Here's how the part is built. I have some questions about the finished solid (model axes, mm). A direction names the side the tool comes from. Round coordinates to 2 decimals unless told otherwise and drop trailing zeros. Loops run counter-clockwise (first coordinate to the right, second up) from the corner with the lowest first, then second, coordinate; pieces in that order, holes last. Notation, with made-up numbers: (-32, 38.5) -> (12, 38.5) arc R21 cw to (12, 64.5) -> close; hole circle Ø9 at (35.25, 25.5). An arc over 180 degrees is marked (long way). Use one line per item in the form item = value. Start each with the question number.
Item 1: If we section it at D-D (x = 25.5): Write out the boundary of the cut face in (y, z).
Item 2: Thinking about a two-plate mould opening in Z: for faces 4 (the face through (-11.265, 97.072, 2.556)), 5 (the face through (-0.2, -0.4, 10.16)), 6 (the face through (-3, 0, 0)), which applies, released by +Z, released by -Z, zero draft, split by the parting line, or undercut?
Item 3: If we section it at C-C (y = -102.5): Write out the boundary of the cut face in (x, z) (3 decimals).
Item 4: For faces 1 (the face through (0, 82.55, 4)), 2 (the face through (0, 0, 8)), 3 (the face through (-28.49, 1.58, 5.01)), which set-ups out of +Z, -Z, +X, -X, +Y, -Y let a thin tool reach every point of the face, with its end or its side?
Item 5: If I drill on L1, parallel to Y at x = -4, z = 8.75; L2, parallel to X at y = 23, z = 5.5; L3, parallel to X at y = 86, z = 7, over which ranges is the centre line in solid material (lowest first)? Write a range as [from, to].
Item 6: If we section it at B-B (y = 76): Write out the boundary of the cut face in (x, z).
Item 7: If we section it at A-A (x = -3): Write out the boundary of the cut face in (y, z) (3 decimals), then the cut area to 3 significant figures.
Item 8: I'm going to push flat-ended pins straight in: pin 1 Ø0.9 at (x, y) = (-2, 89.5) entering from +Z; pin 2 Ø0.6 at (y, z) = (89.5, 2.5) entering from +X; pin 3 Ø16 at (x, y) = (-3, 38) entering from +Z; pin 4 Ø5 at (y, z) = (-54.5, 8) entering from -X. Where does each tip first touch, or does it pass through?
```python
from build123d import *

# Parameters (mm, degrees)
F1_DEPTH     = 7.62
F2_W         = 26.67
F2_H         = 5.08
F3_DEPTH     = 0.508
F5_DEPTH     = 7.62
F7_DEPTH     = 25.4
F8_T1_DEPTH  = 39.5884897473
F8_T3_DEPTH  = 43.1891092466
F8_T5_DEPTH  = 15.7316119842
F8_T10_DEPTH = 21.2484768612
F8_T15_DEPTH = 21.2484768612
F8_T20_DEPTH = 21.2484768612
F8_T25_DEPTH = 21.2484768612
F10_DEPTH    = 10.16
F12_DEPTH    = 3.175
F13_C1_SIZE2 = 5.08
F13_C1_SIZE  = 2.54
F13_C2_SIZE2 = 2.54
F13_C2_SIZE  = 5.08


# Not quite as in the source:
# - a fillet or chamfer that OpenCascade refuses, or shapes differently, is made with other operations: its cross-section is extruded or revolved along the edge and cut away or added


with BuildPart() as f1:
    # F0 (on Top) → F1 (new body)
    with BuildSketch(Plane.XY):
        Polygon((-15.875, 88.9), (-12.7, 0), (12.7, 0), (15.875, 88.9), align=None)
        Polygon((-6.5727372599, 6.35), (-9.2941658314, 82.55), (9.2941658314, 82.55), (6.5727372599, 6.35), align=None, mode=Mode.SUBTRACT)
    extrude(amount=F1_DEPTH)

    # F2 (on face) → F3 (join)
    with BuildSketch(Plane(origin=(0, 88.9, 0), x_dir=(-1, 0, 0), z_dir=(0, 1, 0))):
        with Locations((0, 2.54)):
            Rectangle(F2_W, F2_H)
    extrude(amount=F3_DEPTH)

    # F4 (on Top) → F5 (join, through all)
    with BuildSketch(Plane.XY):
        Polygon((-6.35, 105.2430003945), (-15.875, 89.408), (15.875, 89.408), (6.35, 105.2430003945), align=None)
    extrude(amount=F5_DEPTH)

    # F6 (on Right) → F7 (cut, symmetric)
    with BuildSketch(Plane.YZ):
        Polygon((105.2430003945, 7.62), (89.408, 7.62), (105.2430003945, 1.27), align=None)
    extrude(amount=F7_DEPTH, both=True, mode=Mode.SUBTRACT)

    # F8: chamfer of 1.524 on 6 edges, made by hand

    # F8_s2 → F8_t1 (cut)
    with BuildSketch(Plane.YZ.offset(-19.7942448737)):
        Polygon((88.9, 6.096), (87.376, 7.62), (88.9, 7.62), align=None)
    extrude(amount=F8_T1_DEPTH, mode=Mode.SUBTRACT)

    # F8_s4 → F8_t3 (cut)
    with BuildSketch(Plane.YZ.offset(-21.5945546233)):
        Polygon((89.408, 5.3668893881), (91.4992312711, 6.7813944907), (89.408, 7.62), align=None)
    extrude(amount=F8_T3_DEPTH, mode=Mode.SUBTRACT)

    # F8_s6 → F8_t5 (cut)
    with BuildSketch(Plane.XY.offset(-4.0558059921)):
        Polygon((14.2955997995, 88.9), (15.8186287896, 87.3216061075), (15.875, 88.9), align=None)
        Polygon((-14.2955997995, 88.9), (-15.8186287896, 87.3216061075), (-15.875, 88.9), align=None)
    extrude(amount=F8_T5_DEPTH, mode=Mode.SUBTRACT)


with BuildPart() as f8_tool8:
    # F8_s9 → F8_t10 (new body)
    with BuildSketch(Plane.XY.offset(-6.8142384306)):
        Polygon((13.1798265815, 89.408), (14.4857717649, 91.7175464201), (15.875, 89.408), align=None)
    extrude(amount=F8_T10_DEPTH)

    split(bisect_by=Plane.YZ.offset(13.335), keep=Keep.TOP)


with BuildPart() as f1_1:
    add(f1.part)

    # F8_t7: cut F8_tool8
    add(f8_tool8.part, mode=Mode.SUBTRACT)


with BuildPart() as f8_tool13:
    # F8_s14 → F8_t15 (new body)
    with BuildSketch(Plane.XY.offset(-6.8142384306)):
        Polygon((13.1798265815, 89.408), (14.4857717649, 91.7175464201), (15.875, 89.408), align=None)
    extrude(amount=F8_T15_DEPTH)

    split(bisect_by=Plane.XY.offset(5.08), keep=Keep.TOP)


with BuildPart() as f1_2:
    add(f1_1.part)

    # F8_t12: cut F8_tool13
    add(f8_tool13.part, mode=Mode.SUBTRACT)


with BuildPart() as f8_tool18:
    # F8_s19 → F8_t20 (new body)
    with BuildSketch(Plane.XY.offset(-6.8142384306)):
        Polygon((-14.4857717649, 91.7175464201), (-13.1798265815, 89.408), (-15.875, 89.408), align=None)
    extrude(amount=F8_T20_DEPTH)

    split(bisect_by=Plane.YZ.offset(-13.335), keep=Keep.BOTTOM)


with BuildPart() as f1_3:
    add(f1_2.part)

    # F8_t17: cut F8_tool18
    add(f8_tool18.part, mode=Mode.SUBTRACT)


with BuildPart() as f8_tool23:
    # F8_s24 → F8_t25 (new body)
    with BuildSketch(Plane.XY.offset(-6.8142384306)):
        Polygon((-14.4857717649, 91.7175464201), (-13.1798265815, 89.408), (-15.875, 89.408), align=None)
    extrude(amount=F8_T25_DEPTH)

    split(bisect_by=Plane.XY.offset(5.08), keep=Keep.TOP)


with BuildPart() as f1_4:
    add(f1_3.part)

    # F8_t22: cut F8_tool23
    add(f8_tool23.part, mode=Mode.SUBTRACT)

    # F9 (on Top) → F10 (join)
    with BuildSketch(Plane.XY):
        with BuildLine():
            Line((22.2250049976, 0), (-22.2250049976, 0))
            ThreePointArc((-22.2250049976, 0), (-28.5750049976, 1.626602675), (-33.360963964, 6.1057692308))
            Line((-33.360963964, 6.1057692308), (-35.0741884204, 5.0131183432))
            ThreePointArc((-35.0741884204, 5.0131183432), (-29.5519258835, -0.155151961), (-22.225, -2.032))
            Line((-22.225, -2.032), (22.225, -2.032))
            ThreePointArc((22.225, -2.032), (29.5519258835, -0.155151961), (35.0741884204, 5.0131183432))
            Line((35.0741884204, 5.0131183432), (33.360963964, 6.1057692308))
            ThreePointArc((33.360963964, 6.1057692308), (28.5750049976, 1.626602675), (22.2250049976, 0))
        make_face()
    extrude(amount=F10_DEPTH)

    # F11 (on Top) → F12 (join)
    with BuildSketch(Plane.XY):
        with BuildLine():
            Line((12.7, -2.032), (-12.7, -2.032))
            Line((-12.7, -2.032), (-11.3907730168, -16.6665786134))
            ThreePointArc((-11.3907730168, -16.6665786134), (-7.6578884737, -23.408271606), (-10.1348339359, -30.7055034507))
            Line((-10.1348339359, -30.7055034507), (0, -143.9929821467))
            Line((0, -143.9929821467), (10.1348339359, -30.7055034507))
            ThreePointArc((10.1348339359, -30.7055034507), (7.6578884737, -23.408271606), (11.3907730168, -16.6665786134))
            Line((11.3907730168, -16.6665786134), (12.7, -2.032))
        make_face()
    extrude(amount=F12_DEPTH)

    # F13: chamfer of 2.54 x 5.08 on 4 edges, made by hand

    # F13_c1
    f13_c1_edges = [f1_4.edges().sort_by_distance(p)[0] for p in [
        (-12.0453865084, -9.3492893067, 3.175),
    ]]
    f13_c1_side = f1_4.faces().sort_by_distance((-12.0453865084, -9.3492893067, 3.1242))[0]
    chamfer(f13_c1_edges, length=F13_C1_SIZE, length2=F13_C1_SIZE2, reference=f13_c1_side)

    # F13_c2
    f13_c2_edges = [f1_4.edges().sort_by_distance(p)[0] for p in [
        (6.3424889397, -73.0964499313, 3.175),
    ]]
    f13_c2_side = f1_4.faces().sort_by_distance((6.2918910116, -73.0919233799, 3.175))[0]
    chamfer(f13_c2_edges, length=F13_C2_SIZE, length2=F13_C2_SIZE2, reference=f13_c2_side)


solid = f1_4.part
```
Values found:
q1.outline = (-1.68, 0) -> (0.41, 0) -> (0.41, 10.16) -> (-1.68, 10.16) -> close
q2.face_4 = zero draft
q2.face_5 = released by +Z
q2.face_6 = released by -Z
q3.outline = (-3.712, 0) -> (3.712, 0) -> (3.712, 0.635) -> (0, 2.484) -> (-3.712, 0.635) -> close
q4.face_1 = +Z, -Z
q4.face_2 = +Z
q4.face_3 = +Z, -Z, +Y
q5.L1 = [-2.03, 0]
q5.L2 = [-13.52, -7.17], [7.17, 13.52]
q5.L3 = [-15.77, 15.77]
q6.outline = (-15.41, 0) -> (-9.06, 0) -> (-9.06, 7.62) -> (-15.41, 7.62) -> close; (9.06, 0) -> (15.41, 0) -> (15.41, 7.62) -> (9.06, 7.62) -> close
q7.outline = (-110.459, 0) -> (6.35, 0) -> (6.35, 7.62) -> (0, 7.62) -> (0, 10.16) -> (-2.032, 10.16) -> (-2.032, 3.175) -> (-53.448, 3.175) -> (-110.459, 0.635) -> close; (82.55, 0) -> (105.243, 0) -> (105.243, 1.27) -> (91.499, 6.781) -> (89.408, 5.367) -> (89.408, 5.08) -> (88.9, 5.08) -> (88.9, 6.096) -> (87.376, 7.62) -> (82.55, 7.62) -> close
q7.area = 459 mm2
q8.pin_1 = 5.73
q8.pin_2 = 13.4
q8.pin_3 = 7.62
q8.pin_4 = through
